Here's the drawing with two shaded views (mm, measured from the low corner). I have some questions. A direction names the side the tool comes from. Round coordinates to 2 decimals unless told otherwise and drop trailing zeros. Write each loop counter-clockwise with the first axis right and the second up, starting at its lowest first coordinate (ties: lowest second). Pieces come first, ordered by that corner, then holes. Notation, with made-up numbers: (40, 2.5) -> (61, 2.5) arc R23 cw to (61, 20.5) -> close; hole circle Ø7 at (71, 80.25). An arc over 180 degrees is marked (long way). Use CSV: the item, a comma, the result in double quotes.
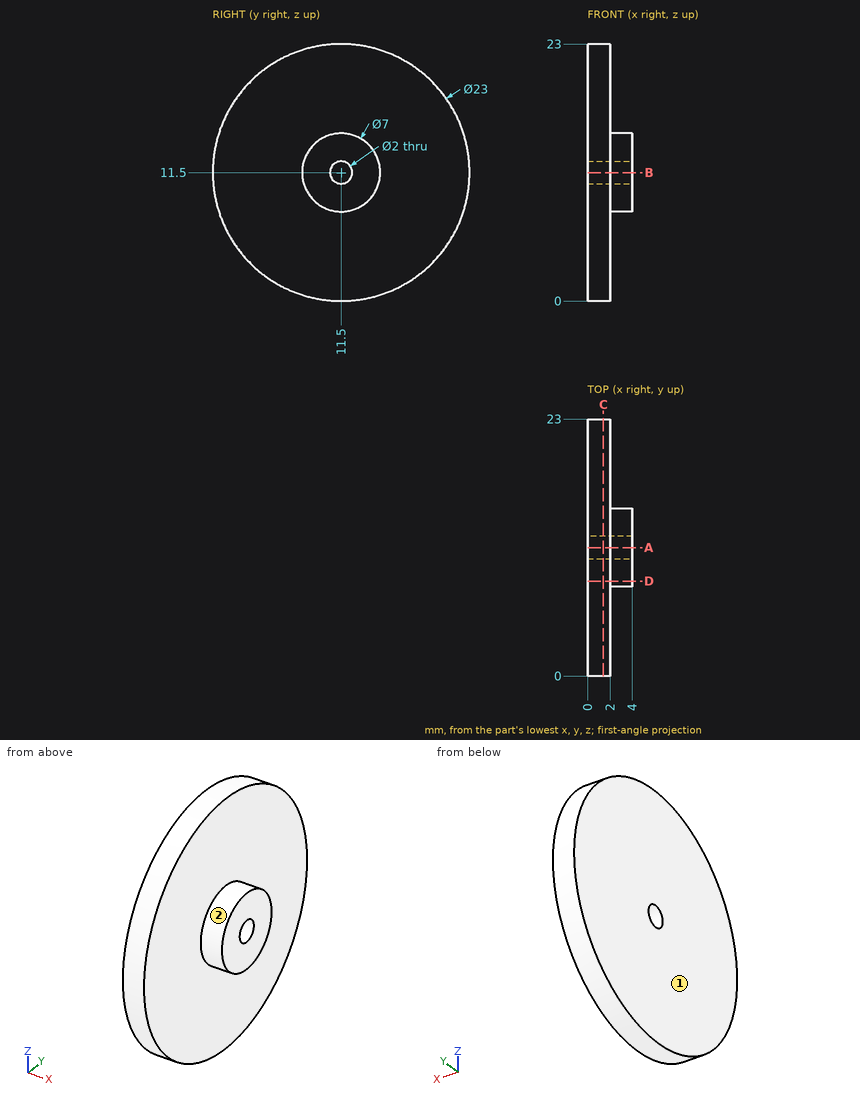
Q1. Please list where these lines run through material, in increasing order: probe 1 along Z at (x, y) = (1.45, 11.5); probe 2 along X at (y, z) = (7, 6); probe 3 along Y at (x, z) = (0.4, 9.25).
Resolved:
probe 1,"z = 0 to 10.5, 12.5 to 23"
probe 2,"x = 0 to 2"
probe 3,"y = 0.22 to 22.78"
Q2. On a 3-axis mill with a long thin cutter (end or side, diameter ignored), from which of +Z, -Z, +X, -X, +Y, -Y can I reach the whole of each face in a straight line? I mean the marked faces 1 and 2. Say none if no direction works.
Resolved:
face 1,"+Z, -Z, -X, +Y, -Y"
face 2,"+X"
Q3. Will this pin go through, and if not, where does the flat tip stop? P1, Ø2.5, axis at y = 11.5, z = 11.5, coming from the -X side.
Resolved:
P1,"stops at x = 0"
Q4. Suppose I cut it at A-A (y = 11.5). Write out the boundary of the cut face in (x, z), and give its area (3 significant figures).
Resolved:
outline,"(0, 0) -> (2, 0) -> (2, 8) -> (4, 8) -> (4, 10.5) -> (0, 10.5) -> close; (0, 12.5) -> (4, 12.5) -> (4, 15) -> (2, 15) -> (2, 23) -> (0, 23) -> close"
area,"52.0 mm^2"
Q5. Suppose I cut it at C-C (x = 1.4). Write out the boundary of the cut face in (y, z), and give its area (3 significant figures).
Resolved:
outline,"circle Ø23 at (11.5, 11.5); hole circle Ø2 at (11.5, 11.5)"
area,"412 mm^2"
Q6. Suppose I cut it at D-D (y = 8.5). Write out the boundary of the cut face in (x, z).
Resolved:
outline,"(0, 0.4) -> (2, 0.4) -> (2, 9.7) -> (4, 9.7) -> (4, 13.3) -> (2, 13.3) -> (2, 22.6) -> (0, 22.6) -> close"
